Geometry check sheet. Reference: the model listing, model coordinates, mm. A direction names the side the tool comes from. Give positions to 0.01 mm unless a question says otherwise; leave off trailing zeros. Write each loop counter-clockwise with the first axis right and the second up, starting at its lowest first coordinate (ties: lowest second). Pieces come first, ordered by that corner, then holes. Notation, with made-up numbers: (-18, 29.25) - (18, 29.25) arc R16 ccw to (18, 35.25) - close; hole circle Ø4 at (-19, 49). An arc over 180 degrees is marked (long way). Use a Markdown table: item, result.
```python
from build123d import *

# Parameters (mm, degrees)
SKETCH_1_W          = 80
SKETCH_1_H          = 70
EXTRUDE_1_DEPTH     = 5
EXTRUDE_2_DEPTH     = 20
SKETCH_3_R          = 1.75
CUT_EXTRUDE_1_DEPTH = 85.728979694
SKETCH_4_R          = 1.75
CUT_EXTRUDE_2_DEPTH = 63.497999968
SKETCH_5_R          = 2.25
CUT_EXTRUDE_3_DEPTH = 57.789083458


with BuildPart() as part:
    # ｽｹｯﾁ1 → ﾎﾞｽ - 押し出し1 (new body)
    with BuildSketch(Plane.XY):
        Rectangle(SKETCH_1_W, SKETCH_1_H)
    extrude(amount=EXTRUDE_1_DEPTH)

    # ｽｹｯﾁ2 → ﾎﾞｽ - 押し出し2 (add)
    with BuildSketch(Plane.XY.offset(5)):
        Polygon((-30, -3), (-21, -3), (-21, -6), (-33, -6), (-33, 6), (-30, 6), align=None)
        Polygon((21, -3), (21, -6), (33, -6), (33, 6), (30, 6), (30, -3), align=None)
    extrude(amount=EXTRUDE_2_DEPTH)

    # ｽｹｯﾁ3 → ｶｯﾄ - 押し出し1 (cut, through all)
    with BuildSketch(Plane(origin=(33, 0, 0), x_dir=(0, 0, -1), z_dir=(1, 0, 0))):
        with Locations(Location((-10, 1.5, 0), (0, 0, 90))):
            Circle(SKETCH_3_R)
        with Locations(Location((-20, 1.5, 0), (0, 0, 90))):
            Circle(SKETCH_3_R)
    extrude(amount=-CUT_EXTRUDE_1_DEPTH, mode=Mode.SUBTRACT)

    # ｽｹｯﾁ4 → ｶｯﾄ - 押し出し2 (cut, through all)
    with BuildSketch(Plane.XZ.offset(6)):
        with Locations((25.5, 10)):
            Circle(SKETCH_4_R)
        with Locations((25.5, 20)):
            Circle(SKETCH_4_R)
        with Locations((-25.5, 10)):
            Circle(SKETCH_4_R)
        with Locations((-25.5, 20)):
            Circle(SKETCH_4_R)
    extrude(amount=-CUT_EXTRUDE_2_DEPTH, mode=Mode.SUBTRACT)

    # ｽｹｯﾁ5 → ｶｯﾄ - 押し出し3 (cut, through all)
    with BuildSketch(Plane.XY.offset(5)):
        with Locations((0, 22.5)):
            Circle(SKETCH_5_R)
        with Locations((19.485571585, -11.25)):
            Circle(SKETCH_5_R)
        with Locations((-19.485571585, -11.25)):
            Circle(SKETCH_5_R)
    extrude(amount=-CUT_EXTRUDE_3_DEPTH, mode=Mode.SUBTRACT)


solid = part.part
```
1) Depth check by flat-ended pin: P1, Ø6, axis at y = 1, z = 10.5, coming from the -X side; P2, Ø9.5, axis at x = 28, z = 13, coming from the -Y side; P3, Ø1, axis at x = 17.5, y = 0, coming from the -Z side; P4, Ø8, axis at y = 7, z = 18, coming from the +X side. Enter the tip coordinate at first touch or a pass-through.
Working result:
| item | result |
|---|---|
| P1 | stops at x = -33 |
| P2 | stops at y = -6 |
| P3 | stops at z = 0 |
| P4 | stops at x = 33 |
2) Section check C-C on z = 20. Record the boundary of the cut face in (x, y), then the cut area to 3 significant figures.
Working result:
| item | result |
|---|---|
| outline | (-33, -6) - (-27.25, -6) - (-27.25, -3) - (-30, -3) - (-30, -0.25) - (-33, -0.25) - close; (-33, 3.25) - (-30, 3.25) - (-30, 6) - (-33, 6) - close; (-23.75, -6) - (-21, -6) - (-21, -3) - (-23.75, -3) - close; (21, -6) - (23.75, -6) - (23.75, -3) - (21, -3) - close; (27.25, -6) - (33, -6) - (33, -0.25) - (30, -0.25) - (30, -3) - (27.25, -3) - close; (30, 3.25) - (33, 3.25) - (33, 6) - (30, 6) - close |
| area | 84.0 mm² |
3) Section check D-D on y = 1.5. Record the boundary of the cut face in (x, z).
Working result:
| item | result |
|---|---|
| outline | (-40, 0) - (40, 0) - (40, 5) - (33, 5) - (33, 8.25) - (30, 8.25) - (30, 5) - (-30, 5) - (-30, 8.25) - (-33, 8.25) - (-33, 5) - (-40, 5) - close; (-33, 11.75) - (-30, 11.75) - (-30, 18.25) - (-33, 18.25) - close; (-33, 21.75) - (-30, 21.75) - (-30, 25) - (-33, 25) - close; (30, 11.75) - (33, 11.75) - (33, 18.25) - (30, 18.25) - close; (30, 21.75) - (33, 21.75) - (33, 25) - (30, 25) - close |
4) Section check A-A on x = 25.5. Record the boundary of the cut face in (y, z), then the cut area to 3 significant figures.
Working result:
| item | result |
|---|---|
| outline | (-35, 0) - (35, 0) - (35, 5) - (-3, 5) - (-3, 8.25) - (-6, 8.25) - (-6, 5) - (-35, 5) - close; (-6, 11.75) - (-3, 11.75) - (-3, 18.25) - (-6, 18.25) - close; (-6, 21.75) - (-3, 21.75) - (-3, 25) - (-6, 25) - close |
| area | 389 mm² |
5) Set-up check for faces 5 (the cylindrical face through (24.21, -4.52, 21.18)), 6 (the flat face through (21, -4, 15)), 7 (the flat face through (26, -3, 15)), 8 (the flat face through (27, -6, 15)), 9 (the flat face through (32, 6, 15)): record each of +Z, -Z, +X, -X, +Y, -Y from which the full face is reachable in a straight line by a thin tool's end or side.
Working result:
| item | result |
|---|---|
| face 5 | +Y, -Y |
| face 6 | +Z, +Y, -Y |
| face 7 | +Z, +Y |
| face 8 | +Z, +X, -X, -Y |
| face 9 | +Z, +X, -X, +Y |
6) Mould release check, pull along X, two halves, no side actions. Record for faces 1 (the flat face through (-33, 0, 15)), 2 (the cylindrical face through (-27.25, -4.52, 10.08)), 3 (the flat face through (-21, -4, 15)), 4 (the flat face through (-32, 6, 15)): pulls with the +X half, pulls with the -X half, needs draft (parallel to the pull), parting line crosses it, or undercut.
Working result:
| item | result |
|---|---|
| face 1 | pulls with the -X half |
| face 2 | undercut |
| face 3 | undercut |
| face 4 | needs draft |
7) Material ranges on L1, parallel to Z at x = -25.5, y = -4.1; L2, parallel to X at y = -3.5, z = 10.5; L3, parallel to Y at x = 0, z = 1.45, recorded low to high. Write a range as from..to.
Working result:
| item | result |
|---|---|
| L1 | z = 0..8.25, 11.75..18.25, 21.75..25 |
| L2 | x = -33..-27.18, -23.82..-21, 21..23.82, 27.18..33 |
| L3 | y = -35..20.25, 24.75..35 |
8) Section check B-B on y = 22.5. Record the boundary of the cut face in (x, z), then the cut area to 4 significant figures.
Working result:
| item | result |
|---|---|
| outline | (-40, 0) - (-2.25, 0) - (-2.25, 5) - (-40, 5) - close; (2.25, 0) - (40, 0) - (40, 5) - (2.25, 5) - close |
| area | 377.5 mm² |
